Autodesk Inventor part; units mm, degrees
ref_plane "YZ Plane" through (0, 0, 0) normal (1, 0, 0) x (0, 1, 0)
ref_plane "XZ Plane" through (0, 0, 0) normal (0, 1, 0) x (-1, 0, 0)
ref_plane "XY Plane" through (0, 0, 0) normal (0, 0, 1) x (1, 0, 0)
sketch "Sketch1" plane through (0, 0, 0) normal (0, 0, 1) x (1, 0, 0)
  line L0 (-2.7585, 21.5) -> (79.762, 21.5)
  line L1 (79.762, 23.5) -> (79.762, 25.5)
  line L2 (79.762, 25.5) -> (-2.7585, 25.5)
  line L3 (-2.7585, 25.5) -> (-2.7585, 23.5)
  line L4 (-2.7585, 21.5) -> (-4.7585, 21.5)
  line L5 (-4.7585, 21.5) -> (-4.7585, 23.5)
  line L6 (-4.7585, 23.5) -> (-2.7585, 23.5)
  line L7 (-2.7585, 23.5) -> (-2.7585, 21.5)
  line L8 (79.762, 25.5) -> (-2.7585, 25.5)
  line L9 (81.762, 23.5) -> (79.762, 23.5)
  line L10 (79.762, 21.5) -> (81.762, 21.5)
  line L11 (81.762, 21.5) -> (81.762, 23.5)
  point P0 (0, 0)
  point P1 (2.8, 2)
  dimension "d0" = 4
  dimension "d1" = 2
  dimension "d2" = 2
extrude "Extrusion1" add sketch "Sketch1" along normal blind 128.3462
sketch "Sketch3" plane through (-4.7585, 21.5, 0) normal (0, -1, 0) x (1, 0, 0)
  line L0 (0, 128.3462) -> (86.5205, 128.3462)
  arc A0 (3.175, 128.3462) -> (0, 125.1712) centre (3.175, 125.1712) ccw
  arc A1 (86.5205, 123.3462) -> (81.5205, 128.3462) centre (81.5205, 123.3462) ccw
  line L1 (0, 0) -> (0, 128.3462)
  line L2 (0, 128.3462) -> (3.175, 128.3462)
  line L3 (0, 128.3462) -> (0, 125.1712)
  line L4 (81.5205, 128.3462) -> (86.5205, 128.3462)
  line L5 (86.5205, 128.3462) -> (86.5205, 123.3462)
  point P0 (4.7585, 0)
  dimension "d5" = 3.175
  dimension "d6" = 5
extrude "Extrusion2" cut sketch "Sketch3" along normal mid plane 128.3462
sketch "Sketch4" plane through (79.762, 23.5, 127.3462) normal (0, 1, 0) x (1, 0, 0)
  line L0 (-84.5205, 127.3462) -> (-84.5205, 2.175)
  line L1 (-82.5205, 127.3462) -> (-82.5205, -0.7746)
  line L2 (0, 127.3462) -> (0, 0)
  line L3 (2, 127.3462) -> (2, 4)
  line L4 (2, 127.3462) -> (0, 127.3462)
  line L5 (-82.5205, 127.3462) -> (-84.5205, 127.3462)
  arc A0 (-84.5205, 2.175) -> (-82.5205, -0.7746) centre (-81.3455, 2.175) ccw
  arc A1 (0, 0) -> (2, 4) centre (-3, 4) ccw
  line L6 (-82.5205, 127.3462) -> (-82.5205, -0.7746)
  line L7 (-82.5205, 127.3462) -> (-81.7705, 127.3462)
  line L8 (-81.7705, 127.3462) -> (-81.7705, -1)
  line L9 (-81.7705, -1) -> (-82.5205, -1)
  line L10 (-82.5205, -1) -> (-82.5205, -0.7746)
  line L11 (0, 127.3462) -> (-0.75, 127.3462)
  line L12 (-0.75, 127.3462) -> (-0.75, -1)
  line L13 (-0.75, -1) -> (0, -1)
  line L14 (0, -1) -> (0, 0)
  point P0 (-79.762, 127.3462)
  dimension "d9" = 0.75
  dimension "d10" = 0.75
extrude "Extrusion3" cut sketch "Sketch4" against normal blind 0.75 and the other way blind 25.4
sketch "Sketch5" plane through (-4.7585, 21.5, 0) normal (0, -1, 0) x (1, 0, 0)
  line L0 (33.02, 122.7582) -> (53.5005, 122.7582)
  line L1 (53.5005, 122.7582) -> (53.5005, 119.7582)
  line L2 (53.5005, 119.7582) -> (33.02, 119.7582)
  line L3 (33.02, 119.7582) -> (33.02, 122.7582)
  line L4 (3.175, 128.3462) -> (81.5205, 128.3462)
  line L5 (86.5205, 0) -> (86.5205, 123.3462)
  line L6 (0, 0) -> (0, 125.1712)
  point P0 (4.7585, 0)
  dimension "d15" = 5.588
  dimension "d16" = 33.02
  dimension "d17" = 33.02
  dimension "d18" = 3
extrude "Extrusion4" add sketch "Sketch5" along normal blind 1
sketch "Sketch6" plane through (-4.7585, 21.5, 0) normal (0, -1, 0) x (1, 0, 0)
  line L0 (0, 0) -> (0, 125.1712)
  line L1 (83.7705, 127.8113) -> (83.7705, 0)
  line L2 (83.7705, 0) -> (2.75, 0)
  line L3 (2.75, 0) -> (2.75, 128.3176)
  arc A0 (3.175, 128.3462) -> (2.75, 128.3176) centre (3.175, 125.1712) ccw
  line L4 (81.5205, 128.3462) -> (3.175, 128.3462)
  arc A1 (83.7705, 127.8113) -> (81.5205, 128.3462) centre (81.5205, 123.3462) ccw
  line L5 (6.75, 70.3822) -> (6.75, 114.3462)
  line L6 (0, 0) -> (86.5205, 0)
  line L7 (6.75, 114.3462) -> (79.7705, 114.3462)
  line L8 (79.7705, 114.3462) -> (79.7705, 0)
  line L9 (79.7705, 0) -> (6.75, 0)
  line L10 (6.75, 0) -> (6.75, 114.3462)
  point P0 (4.7585, 0)
  dimension "d21" = 4
  dimension "d22" = 14
  dimension "d23" = 4
extrude "Extrusion5" cut sketch "Sketch6" against normal blind 1.75 contours L2 L10 L5 L7 L8
properties part number "Capstone Calculator Back Cover"
Can you work these out from the model? Positions are in its coordinate system, mm. A direction names the side the tool comes from. Give positions to 0.01 mm unless a question says otherwise; leave off trailing zeros. Loops run counter-clockwise (first coordinate to the right, second up) from the corner with the lowest first, then second, coordinate; pieces in that order, holes last. Notation, with made-up numbers: (70.25, 69) - (107.25, 69) arc R20 ccw to (107.25, 76) - close; hole circle Ø5 at (14, 51.25). An arc over 180 degrees is marked (long way). Answer as a JSON object with one key per item and string values.
Q1. Will these pins go through, and if not, where does the flat tip stop? P1, Ø0.8, axis at y = 23.5, z = 94.5, coming from the +X side; P2, Ø1.4, axis at x = 81, z = 93, coming from the +Y side; P3, Ø3, axis at y = 24.5, z = 61, coming from the -X side.
Geometry says:
{"P1": "x = 79.01", "P2": "y = 22.75", "P3": "x = -2.01"}
Q2. Imagine slicing it at A-A on x = 35.5. Write out the boundary of the cut face in (y, z), plus the area to 3 significant figures.
Geometry says:
{"outline": "(20.5, 119.76) - (21.5, 119.76) - (21.5, 114.35) - (23.25, 114.35) - (23.25, 0) - (25.5, 0) - (25.5, 128.35) - (21.5, 128.35) - (21.5, 122.76) - (20.5, 122.76) - close", "area": "316 mm²"}
Q3. Imagine slicing it at D-D on x = 23. Write out the boundary of the cut face in (y, z).
Geometry says:
{"outline": "(21.5, 114.35) - (23.25, 114.35) - (23.25, 0) - (25.5, 0) - (25.5, 128.35) - (21.5, 128.35) - close"}
Q4. Imagine slicing it at B-B on z = 54.5. Write out the boundary of the cut face in (x, y).
Geometry says:
{"outline": "(-4.76, 21.5) - (1.99, 21.5) - (1.99, 23.25) - (75.01, 23.25) - (75.01, 21.5) - (81.76, 21.5) - (81.76, 22.75) - (79.01, 22.75) - (79.01, 25.5) - (-2.01, 25.5) - (-2.01, 22.75) - (-4.76, 22.75) - close"}
Q5. If I drill on L1, parallel to X at y = 21.75, z = 26; L2, parallel to X at y = 23.05, z = 38.5; L3, parallel to X at y = 23.4, z = 72, over which ranges is the centre line in solid material (lowest first)?
Geometry says:
{"L1": "-4.76 to 1.99, 75.01 to 81.76", "L2": "-2.01 to 1.99, 75.01 to 79.01", "L3": "-2.01 to 79.01"}
Q6. If we mould it in two halves opening along X, with no side actions, what happens to faces 1 (the flat face through (79.012, 24, 63)), 2 (the flat face through (38, 21.5, 116)), 3 (the cylindrical face through (-3.433, 22.195, 127.752)), 4 (the flat face through (38, 23.25, 58))? For each: pulls with the +X half, pulls with the -X half, needs draft (parallel to the pull), parting line crosses it, or undercut.
Geometry says:
{"face 1": "pulls with the +X half", "face 2": "needs draft", "face 3": "pulls with the -X half", "face 4": "undercut"}
Q7. Which directions (+Z, -Z, +X, -X, +Y, -Y) give clear straight access to the entire face, cutting with the end or side of a thin tool? Please do faces 5 (the flat face through (80, 22.75, 63)), 6 (the flat face through (-2.009, 24, 63)), 7 (the flat face through (38, 24, 0)).
Geometry says:
{"face 5": "+Z, -Z, +X, +Y", "face 6": "+Z, -Z, -X, +Y", "face 7": "-Z, +X, -X, +Y, -Y"}
